from build123d import *

# Parameters (mm, degrees)
SKETCH1_W           = 25.4
SKETCH1_H           = 50.8
BOSS_EXTRUDE1_DEPTH = 127
SHELL1_T            = -1.5875
SKETCH2_R           = 2.4892
CUT_EXTRUDE1_DEPTH  = 140.121529606
SKETCH3_R           = 2.4892
CUT_EXTRUDE2_DEPTH  = 140.121529606


with BuildPart() as part:
    # Sketch1 → Boss-Extrude1 (new body)
    with BuildSketch(Plane.XY):
        with Locations((12.7, 25.4)):
            Rectangle(SKETCH1_W, SKETCH1_H)
    extrude(amount=BOSS_EXTRUDE1_DEPTH)

    # Shell1
    shell1_openings = [part.faces().sort_by_distance(p)[0] for p in [
        (12.7, 25.4, 127),
        (12.7, 25.4, 0),
    ]]
    offset(amount=SHELL1_T, openings=shell1_openings, kind=Kind.INTERSECTION)

    # Sketch2 → Cut-Extrude1 (cut, through all)
    with BuildSketch(Plane.ZY):
        with Locations(Location((12.7, 12.7, 0), (0, 0, 270))):
            Circle(SKETCH2_R)
        with Locations(Location((38.1, 12.7, 0), (0, 0, 270))):
            Circle(SKETCH2_R)
        with Locations(Location((63.5, 12.7, 0), (0, 0, 270))):
            Circle(SKETCH2_R)
        with Locations(Location((88.9, 12.7, 0), (0, 0, 270))):
            Circle(SKETCH2_R)
        with Locations(Location((114.3, 12.7, 0), (0, 0, 270))):
            Circle(SKETCH2_R)
        with Locations(Location((38.1, 38.1, 0), (0, 0, 270))):
            Circle(SKETCH2_R)
        with Locations(Location((63.5, 38.1, 0), (0, 0, 270))):
            Circle(SKETCH2_R)
        with Locations(Location((88.9, 38.1, 0), (0, 0, 270))):
            Circle(SKETCH2_R)
        with Locations(Location((114.3, 38.1, 0), (0, 0, 270))):
            Circle(SKETCH2_R)
        with Locations(Location((12.7, 38.1, 0), (0, 0, 270))):
            Circle(SKETCH2_R)
    extrude(amount=-CUT_EXTRUDE1_DEPTH, mode=Mode.SUBTRACT)

    # Sketch3 → Cut-Extrude2 (cut, through all)
    with BuildSketch(Plane(origin=(0, 50.8, 0), x_dir=(1, 0, 0), z_dir=(0, 1, 0))):
        with Locations(Location((12.7, -12.7, 0), (0, 0, 270))):
            Circle(SKETCH3_R)
        with Locations(Location((12.7, -38.1, 0), (0, 0, 270))):
            Circle(SKETCH3_R)
        with Locations(Location((12.7, -63.5, 0), (0, 0, 270))):
            Circle(SKETCH3_R)
        with Locations(Location((12.7, -88.9, 0), (0, 0, 270))):
            Circle(SKETCH3_R)
        with Locations(Location((12.7, -114.3, 0), (0, 0, 270))):
            Circle(SKETCH3_R)
    extrude(amount=-CUT_EXTRUDE2_DEPTH, mode=Mode.SUBTRACT)


solid = part.part
Verification items for the finished model (mm, model axes). A direction names the side the tool comes from. Give positions to 0.01 mm unless a question says otherwise; leave off trailing zeros. Write each loop counter-clockwise with the first axis right and the second up, starting at its lowest first coordinate (ties: lowest second). Pieces come first, ordered by that corner, then holes. Notation, with made-up numbers: (3.5, -1.5) -> (53.5, -1.5) arc R30 ccw to (53.5, 35.5) -> close; hole circle Ø2 at (-20, 46.25). An arc over 180 degrees is marked (long way). Use CSV: the item, a comma, the result in double quotes.
(1) Sectioned sample at C-C (x = 7.25). Record the cut outline in (y, z), plus the area to 3 significant figures.
Derived:
outline,"(0, 0) -> (1.59, 0) -> (1.59, 127) -> (0, 127) -> close; (49.21, 0) -> (50.8, 0) -> (50.8, 127) -> (49.21, 127) -> close"
area,"403 mm^2"
(2) Material ranges on L1, parallel to Z at x = 24.3, y = 38.1; L2, parallel to X at y = 38, z = 78; L3, parallel to Y at x = 6.75, z = 85, recorded low to high.
Derived:
L1,"z = 0 to 10.21, 15.19 to 35.61, 40.59 to 61.01, 65.99 to 86.41, 91.39 to 111.81, 116.79 to 127"
L2,"x = 0 to 1.59, 23.81 to 25.4"
L3,"y = 0 to 1.59, 49.21 to 50.8"
(3) Sectioned sample at B-B (z = 45). Record the cut outline in (x, y), plus the area to 3 significant figures.
Derived:
outline,"(0, 0) -> (25.4, 0) -> (25.4, 50.8) -> (0, 50.8) -> close; hole (1.59, 1.59) -> (23.81, 1.59) -> (23.81, 49.21) -> (1.59, 49.21) -> close"
area,"232 mm^2"
(4) Go/stop test with a flat-tipped pin: pin 1 (3 mm diameter, centred on y = 38.1, z = 88.9, fed in from -X). Record where the tip stops, or that it passes through.
Derived:
pin 1,"passes through"
(5) Sectioned sample at A-A (y = 6.5). Record the cut outline in (x, z), plus the area to 3 significant figures.
Derived:
outline,"(0, 0) -> (1.59, 0) -> (1.59, 127) -> (0, 127) -> close; (23.81, 0) -> (25.4, 0) -> (25.4, 127) -> (23.81, 127) -> close"
area,"403 mm^2"
(6) Set-up check for faces 1 (the cylindrical face through (24.6, 38.64, 35.67)), 2 (the flat face through (1.588, 25, 63)): record each of +Z, -Z, +X, -X, +Y, -Y from which the full face is reachable in a straight line by a thin tool's end or side.
Derived:
face 1,"+X, -X"
face 2,"+Z, -Z"
(7) Release check for a two-part mould opening along Y. For faces 3 (the cylindrical face through (24.6, 36.76, 91)), 4 (the cylindrical face through (12.809, 0.805, 61.013)), 5 (the flat face through (23.812, 25, 63)), 6 (the flat face through (15.3, 50.8, 62.6)) record: +Y half, -Y half, draft (parallel to the pull), parting line (faces both ways), or undercut.
Derived:
face 3,"undercut"
face 4,"draft"
face 5,"undercut"
face 6,"+Y half"
(8) Sectioned sample at D-D (z = 114.3). Give the number of separate pieces and of enclosed holes in the cut face, plus the area to 3 significant figures.
Derived:
separate pieces,"6"
enclosed holes,"0"
area,"184 mm^2"
